Design review of the part built by this model. Coordinates are the model's own, in mm. Face numbers are marked on the shaded views. A direction names the side the tool comes from. Coordinates: 2 decimals unless noted, no trailing zeros. Write each loop counter-clockwise with the first axis right and the second up, starting at its lowest first coordinate (ties: lowest second). Pieces come first, ordered by that corner, then holes.
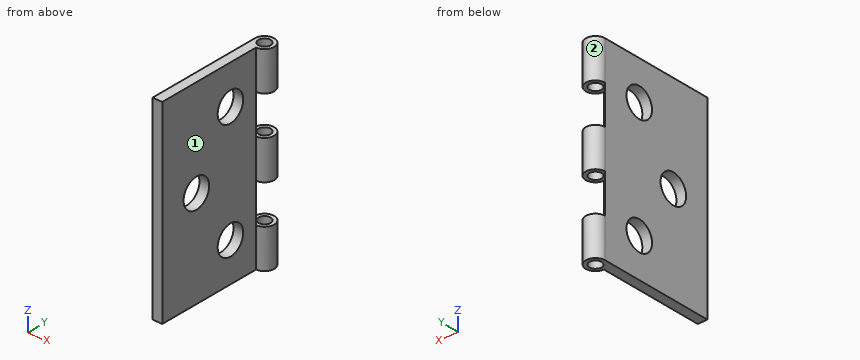
```python
from build123d import *

# Parameters (mm, degrees)
SKETCH1_W           = 50
SKETCH1_H           = 30
SKETCH1_R           = 3.75
BOSS_EXTRUDE1_DEPTH = 2.5
SKETCH3_R           = 2.5
BOSS_EXTRUDE3_DEPTH = 10
SKETCH4_R           = 1.575
CUT_EXTRUDE1_DEPTH  = 50
LPATTERN1_COUNT     = 3
LPATTERN1_PITCH     = 20
CUT_EXTRUDE3_START  = -10
SKETCH5_R           = 2.5
CUT_EXTRUDE3_DEPTH  = 10
CUT_EXTRUDE4_START  = -40
SKETCH5_2_R         = 2.5
CUT_EXTRUDE4_DEPTH  = 10
ESCALA1_SCALE       = 0.5


with BuildPart() as part:
    # Sketch1 → Boss-Extrude1 (new body)
    with BuildSketch(Plane(origin=(0, 0, 0), x_dir=(0, 0, -1), z_dir=(1, 0, 0))):
        with Locations((25, 15)):
            Rectangle(SKETCH1_W, SKETCH1_H)
        with Locations((40, 20)):
            Circle(SKETCH1_R, mode=Mode.SUBTRACT)
        with Locations((25, 10)):
            Circle(SKETCH1_R, mode=Mode.SUBTRACT)
        with Locations((10, 20)):
            Circle(SKETCH1_R, mode=Mode.SUBTRACT)
    extrude(amount=BOSS_EXTRUDE1_DEPTH)

    # Sketch3 → Boss-Extrude3 (add)
    with BuildSketch(Plane(origin=(0, 0, -50), x_dir=(-1, 0, 0), z_dir=(0, 0, -1))):
        with Locations((-2.5, 30)):
            Circle(SKETCH3_R)
    boss_extrude3 = extrude(amount=-BOSS_EXTRUDE3_DEPTH)

    # Sketch4 → Cut-Extrude1 (cut)
    with BuildSketch(Plane(origin=(0, 0, -50), x_dir=(-1, 0, 0), z_dir=(0, 0, -1))):
        with Locations((-2.5, 30)):
            Circle(SKETCH4_R)
    cut_extrude1 = extrude(amount=-CUT_EXTRUDE1_DEPTH, mode=Mode.SUBTRACT)

    # LPattern1: Boss-Extrude3, Cut-Extrude1 ×3
    with Locations(*[(0, 0, i * LPATTERN1_PITCH) for i in range(1, LPATTERN1_COUNT)]):
        add(boss_extrude3)
        add(cut_extrude1, mode=Mode.SUBTRACT)

    # Sketch5 → Cut-Extrude3 (cut)
    with BuildSketch(Plane(origin=(0, 0, -50), x_dir=(-1, 0, 0), z_dir=(0, 0, -1)).offset(CUT_EXTRUDE3_START)):
        with Locations((-2.5, 30)):
            Circle(SKETCH5_R)
    extrude(amount=-CUT_EXTRUDE3_DEPTH, mode=Mode.SUBTRACT)

    # Sketch5<2> → Cut-Extrude4 (cut)
    with BuildSketch(Plane(origin=(0, 0, -50), x_dir=(-1, 0, 0), z_dir=(0, 0, -1)).offset(CUT_EXTRUDE4_START)):
        with Locations((-2.5, 30)):
            Circle(SKETCH5_2_R)
    extrude(amount=CUT_EXTRUDE4_DEPTH, mode=Mode.SUBTRACT)


with BuildPart() as part_1:
    # Escala1: scaled about (0, 0, 0)
    add(part.part.scale(ESCALA1_SCALE))


solid = part_1.part
```
(1) For the marked faces 1 and 2, list the 3-axis set-ups (+Z, -Z, +X, -X, +Y, -Y) from which the entire face can be reached by the end or side of a thin tool; tool diameter is ignored.
(2) Consider section A-A (z = -12.5). State how many separate pieces and enclosed holes the cut face has, plus the area to 3 significant figures.
(3) Consider section B-B (y = 5). Give the boundary of the cut face in (x, z) (3 decimals).
(4) Wall thickness on line 1 (X direction, y = 15, z = -13.25); line 2 (Z direction, x = 0.8, y = 11.5) (3 decimals); line 3 (X direction, y = 7.75, z = -20.5): over which ranges is each line inside the solid? List them lowest first.
(5) Insertion check: pin 1 Ø3.5 at (y, z) = (5, -12.5) entering from +X; pin 2 Ø1.5 at (y, z) = (7, -3) entering from +X; pin 3 Ø3 at (y, z) = (14.5, -7.5) entering from +X. Each pin has a flat end and moves straight along its axis. Give the tip position at first contact, or say it passes through.
(6) Consider section D-D (z = -15.5). Give the boundary of the cut face in (x, y).
(7) Consider section C-C (y = 9). Give the boundary of the cut face in (x, z), plus the area to 3 significant figures.
Results:
1. face 1: +Z, -Z, +X, -Y
1. face 2: +Z, -Z
2. separate pieces: 2
2. enclosed holes: 1
2. area: 15.8 mm2
3. outline: (0, -25) - (1.25, -25) - (1.25, -14.375) - (0, -14.375) - close; (0, -10.625) - (1.25, -10.625) - (1.25, 0) - (0, 0) - close
4. line 1: x = 0 to 0.46, 2.04 to 2.5
4. line 2: z = -25 to -21.125, -18.875 to -6.125, -3.875 to 0
4. line 3: x = 0 to 1.25
5. pin 1: passes through
5. pin 2: stops at x = 1.25
5. pin 3: stops at x = 1.25
6. outline: (0, 0) - (1.25, 0) - (1.25, 13.75) arc R1.25 cw to (0, 15) - close
7. outline: (0, -25) - (1.25, -25) - (1.25, -21.59) - (0, -21.59) - close; (0, -18.41) - (1.25, -18.41) - (1.25, -6.59) - (0, -6.59) - close; (0, -3.41) - (1.25, -3.41) - (1.25, 0) - (0, 0) - close
7. area: 23.3 mm2
